Check sheet for the modelled part. Datum: model origin and axes. Units: mm. Coordinates: 2 decimals unless noted, no trailing zeros. Loops run counter-clockwise (first coordinate to the right, second up) from the corner with the lowest first, then second, coordinate; pieces in that order, holes last. Notation, with made-up numbers: (26, -1.75) -> (56, -1.75) arc R22 ccw to (56, 17.25) -> close; hole circle Ø1 at (-16, -24.75). An arc over 180 degrees is marked (long way). Use CSV: the item, a comma, the result in double quotes. Start each with the question number.
1. Thickness scan on L1, parallel to Z at x = 12, y = 8.25; L2, parallel to Y at x = -12, z = -1; L3, parallel to X at y = 5.75, z = -4. Record the ranges inside material, lowest first.
2. Sectioned sample at C-C, the plane x = -4. Record the cut outline in (y, z), and give its area (3 significant figures).
3. Sectioned sample at D-D, the plane z = -3. Record the cut outline in (x, y), and give its area (3 significant figures).
4. Sectioned sample at A-A, the plane z = 0. Record the cut outline in (x, y), and give its area (3 significant figures).
5. Gauge pin test, flat end, axial feed: pin 1 (2 mm diameter, centred on x = 12.5, z = 3, fed in from -Y). Record the tip position at first contact, or that the pin passes through.
6. Release check for a two-part mould opening along Y. For faces 1 (the face through (-17, 5, 0)), 2 (the face through (5.31, 4, -0.07)), 3 (the face through (0, 0, 0)), 4 (the face through (0, 10, 0)) record: pulls with the +Y half, pulls with the -Y half, needs draft (parallel to the pull), parting line crosses it, or undercut.
7. Sectioned sample at B-B, the plane y = 5. Record the cut outline in (x, z), and give its area (3 significant figures).
```python
from build123d import *

# Parameters (mm, degrees)
SKETCH_1_W         = 34
SKETCH_1_H         = 10
EXTRUDE_1_DEPTH    = 10
HOLE_WIZARD_M4_1_D = 3.3
HOLE_WIZARD_M4_3_D = 3.3


with BuildPart() as part:
    # 草图1 → 凸台-拉伸1 (new body)
    with BuildSketch(Plane(origin=(0, 0, 0), x_dir=(1, 0, 0), z_dir=(0, 1, 0))):
        Rectangle(SKETCH_1_W, SKETCH_1_H)
    extrude(amount=EXTRUDE_1_DEPTH)

    # M4 螺纹孔1 (through all)
    with Locations(Plane.XY.offset(5)):
        with Locations((4, 5), (-12, 5)):
            Hole(HOLE_WIZARD_M4_1_D / 2)

    # M4 螺纹孔3 (through all)
    with Locations(Plane(origin=(0, 10, 0), x_dir=(1, 0, 0), z_dir=(0, 1, 0))):
        with Locations((-4, 0), (12, 0)):
            Hole(HOLE_WIZARD_M4_3_D / 2)


solid = part.part
```
Completed:
1,L1,"-5 to -1.65, 1.65 to 5"
1,L2,"0 to 3.35, 6.65 to 10"
1,L3,"-17 to -13.47, -10.53 to 2.53, 5.47 to 17"
2,outline,"(0, -5) -> (10, -5) -> (10, -1.65) -> (0, -1.65) -> close; (0, 1.65) -> (10, 1.65) -> (10, 5) -> (0, 5) -> close"
2,area,"67.0 mm²"
3,outline,"(-17, 0) -> (17, 0) -> (17, 10) -> (-17, 10) -> close; hole circle Ø3.3 at (-12, 5); hole circle Ø3.3 at (4, 5)"
3,area,"323 mm²"
4,outline,"(-17, 0) -> (-5.65, 0) -> (-5.65, 10) -> (-17, 10) -> close; (-2.35, 0) -> (10.35, 0) -> (10.35, 10) -> (-2.35, 10) -> close; (13.65, 0) -> (17, 0) -> (17, 10) -> (13.65, 10) -> close; hole circle Ø3.3 at (-12, 5); hole circle Ø3.3 at (4, 5)"
4,area,"257 mm²"
5,pin 1,"y = 0"
6,face 1,"needs draft"
6,face 2,"undercut"
6,face 3,"pulls with the -Y half"
6,face 4,"pulls with the +Y half"
7,outline,"(-17, -5) -> (-13.65, -5) -> (-13.65, 5) -> (-17, 5) -> close; (-10.35, -5) -> (2.35, -5) -> (2.35, 5) -> (-10.35, 5) -> close; (5.65, -5) -> (17, -5) -> (17, 5) -> (5.65, 5) -> close; hole circle Ø3.3 at (-4, 0); hole circle Ø3.3 at (12, 0)"
7,area,"257 mm²"
